Build history of the part. All positions in model axes, mm. A direction names the side the tool comes from. Give positions to 0.01 mm unless a question says otherwise; leave off trailing zeros. Write each loop counter-clockwise with the first axis right and the second up, starting at its lowest first coordinate (ties: lowest second). Pieces come first, ordered by that corner, then holes. Notation, with made-up numbers: M 32.25,-13.5 L 42.25,-13.5 A6 cw 42.25,-6.5 Z; hole C 25,56 d8. An arc over 180 degrees is marked long. Return JSON: item names as keys, results as strings. Group by question number.
Q1. Tool access for faces 1 (the flat face through (-3.944, 2.7, -10.1)), 2 (the flat face through (0, 1.643, -19)), 3 (the flat face through (3.944, 2.7, -10.1)), 4 (the flat face through (-10.499, 2, -15)): list every direction of +Z, -Z, +X, -X, +Y, -Y with a clear straight run to the whole face (end or side of a thin tool).
Q2. Band-saw the part on A-A, the plane y = 3.2. Give the cut face in (x, z).
Q3. Pull direction X, two halves, no side cores. Call faces 5 (the flat face through (10.499, 2, -15)), 6 (the cylindrical face through (6.664, 1.63, -14.967)), 7 (the flat face through (0, 1.643, -12)): +X half, -X half, draft (parallel to the pull), parting line (faces both ways), or undercut.
Q4. Band-saw the part on D-D, the plane z = -17. Count the separate pieces of the cut face and the enclosed holes in it, then the cut area to 3 significant figures.
Q5. Band-saw the part on B-B, the plane z = -9.5. Give the cut face in (x, y).
Q6. Wall check: probe 1 along Y at (x, z) = (-0.75, -12.75); probe 2 along Y at (x, z) = (-8.75, -15.25); probe 3 along Z at (x, y) = (-1, 3.7). Give the ranges that are in metal, low to high.
Q7. Flat gauge pins, fed straight in: pin 1 Ø0.9 at (x, z) = (-3.5, -19) entering from -Y; pin 2 Ø1.5 at (x, z) = (0.5, -14.5) entering from +Y; pin 3 Ø1.1 at (y, z) = (4, -10) entering from -X. Where does each tip first touch, or does it go through?
Q8. Band-saw the part on C-C, the plane x = -0.5. Give the cut face in (y, z).
from build123d import *

# Parameters (mm, degrees)
BOSS_EXTRUDE1_DEPTH        = 23.666666667
SKETCH2_W                  = 25
SKETCH2_H                  = 3.5
BOSS_EXTRUDE2_DEPTH        = 19.666666667
SKETCH3_W                  = 25
SKETCH3_H                  = 3.5
BOSS_EXTRUDE3_DEPTH        = 19.666666667
SKETCH4_W                  = 63
SKETCH4_H                  = 14.75
BOSS_EXTRUDE4_DEPTH        = 0.8
SKETCH5_W                  = 5.25
SKETCH5_H                  = 0.8
CUT_EXTRUDE1_DEPTH         = 72.070387645
F_10_CLEARANCE_HOLE1_D     = 5.5
F_10_CLEARANCE_HOLE1_DEPTH = 43.333333333
HOLE1_AT_2_COUNT           = 2
HOLE1_AT_2_PITCH           = 37
FILLET1_R                  = 0.8
SCALE1_SCALE               = 0.3333


with BuildPart() as part:
    # Sketch1 → Boss-Extrude1 (new body)
    with BuildSketch(Plane(origin=(11.833333333, 0, 0), x_dir=(0, 0, -1), z_dir=(1, 0, 0))):
        with BuildLine():
            Line((31, 3.5), (5.123475383, 3.5))
            ThreePointArc((5.123475383, 3.5), (-3.102418411, 10.041475531), (0, 0))
            Line((0, 0), (31, 0))
            Line((31, 0), (31, 3.5))
        make_face()
    extrude(amount=-BOSS_EXTRUDE1_DEPTH)

    # Sketch2 → Boss-Extrude2 (add)
    with BuildSketch(Plane.ZY.offset(11.833333333)):
        with Locations((-18.5, 1.75)):
            Rectangle(SKETCH2_W, SKETCH2_H)
    extrude(amount=BOSS_EXTRUDE2_DEPTH)

    # Sketch3 → Boss-Extrude3 (add)
    with BuildSketch(Plane(origin=(11.833333333, 0, 0), x_dir=(0, 0, -1), z_dir=(1, 0, 0))):
        with Locations((18.5, 1.75)):
            Rectangle(SKETCH3_W, SKETCH3_H)
    extrude(amount=BOSS_EXTRUDE3_DEPTH)

    # Sketch4 → Boss-Extrude4 (add)
    with BuildSketch(Plane.XZ):
        with Locations((0, -23.625)):
            Rectangle(SKETCH4_W, SKETCH4_H)
    extrude(amount=BOSS_EXTRUDE4_DEPTH)

    # Sketch5 → Cut-Extrude1 (cut, through all)
    with BuildSketch(Plane(origin=(31.5, 0, 0), x_dir=(0, 0, -1), z_dir=(1, 0, 0))):
        with Locations((28.375, -0.4)):
            Rectangle(SKETCH5_W, SKETCH5_H)
    extrude(amount=-CUT_EXTRUDE1_DEPTH, mode=Mode.SUBTRACT)

    # #10 Clearance Hole1
    with Locations(Plane.ZY.offset(11.833333333)):
        with Locations((0, 5.5)):
            Hole(F_10_CLEARANCE_HOLE1_D / 2, depth=F_10_CLEARANCE_HOLE1_DEPTH)

    # Sketch8 → Hole1 (revolve, cut)
    with BuildSketch(Plane(origin=(-18.5, 3.5, -21), x_dir=(0, 0, 1), z_dir=(1, 0, 0))):
        Polygon((0, 0), (0, 4.3), (3.9, 4.3), (3.9, 2.8), (6.5, 0), align=None)
    hole1 = revolve(axis=Axis((-18.5, 9.945314094, -21), (0, -1, 0)), mode=Mode.SUBTRACT)

    # Hole1 at 2: Hole1 ×2
    with Locations(*[(i * HOLE1_AT_2_PITCH, 0, 0) for i in range(1, HOLE1_AT_2_COUNT)]):
        add(hole1, mode=Mode.SUBTRACT)

    # Fillet1
    fillet1_edges = [part.edges().sort_by_distance(p)[0] for p in [
        (0, 3.5, -31),
    ]]
    fillet(fillet1_edges, radius=FILLET1_R)


with BuildPart() as part_1:
    # Scale1: scaled about (0, 2.464609402, -13.752110163)
    add(part.part.scale(SCALE1_SCALE).moved(Location((0, 1.643155088, -9.168531846))))


solid = part_1.part
From the geometry:
{
 "1": {"face 1": "+Z, -X, +Y, -Y", "face 2": "-Z, +X, -X, -Y", "face 3": "+Z, +X, +Y, -Y", "face 4": "+Z, -Z, -X, +Y, -Y"},
 "2": {"outline": "M -3.94,-10.98 L 3.94,-10.98 L 3.94,-10.04 L -3.94,-10.04 Z; M -3.94,-8.29 L 3.94,-8.29 L 3.94,-7.36 L -3.94,-7.36 Z"},
 "3": {"face 5": "+X half", "face 6": "undercut", "face 7": "draft"},
 "4": {"separate pieces": "3", "enclosed holes": "0", "area": "22.4 mm^2"},
 "5": {"outline": "M -3.94,1.64 L 3.94,1.64 L 3.94,2.62 L -3.94,2.62 Z; M -3.94,4.33 L 3.94,4.33 L 3.94,5.28 L -3.94,5.28 Z"},
 "6": {"probe 1": "y = 1.64 to 2.81", "probe 2": "y = 1.38 to 2.81", "probe 3": "z = -10.99 to -10.06, -8.28 to -7.35"},
 "7": {"pin 1": "stops at y = 1.64", "pin 2": "stops at y = 2.81", "pin 3": "stops at x = -3.94"},
 "8": {"outline": "M 1.38,-17.75 L 1.64,-17.75 L 1.64,-19.5 L 2.54,-19.5 A0.27 ccw 2.81,-19.23 L 2.81,-10.88 A1.83 ccw long 1.64,-9.17 L 1.64,-14.58 L 1.38,-14.58 Z; hole C 3.48,-9.17 d1.83"}
}
